```python
from build123d import *

# Parameters (mm, degrees)
SKIZZE1_W                       = 135
SKIZZE1_H                       = 135
SKIZZE1_W_2                     = 131
SKIZZE1_H_2                     = 131
AUFSATZ_LINEAR_AUSTRAGEN1_DEPTH = 18
SKIZZE2_W                       = 135
SKIZZE2_H                       = 135
AUFSATZ_LINEAR_AUSTRAGEN2_DEPTH = 5
SCHNITT_LINEAR_AUSTRAGEN1_DEPTH = 11
SKIZZE4_R                       = 1.75
SKIZZE4_R_2                     = 0.5
SCHNITT_LINEAR_AUSTRAGEN2_DEPTH = 10
FASE1_SIZE                      = 1


with BuildPart() as part:
    # Skizze1 → Aufsatz-Linear austragen1 (new body)
    with BuildSketch(Plane.XY):
        Rectangle(SKIZZE1_W, SKIZZE1_H)
        Rectangle(SKIZZE1_W_2, SKIZZE1_H_2, mode=Mode.SUBTRACT)
    extrude(amount=AUFSATZ_LINEAR_AUSTRAGEN1_DEPTH)

    # Skizze2 → Aufsatz-Linear austragen2 (add)
    with BuildSketch(Plane.XY.offset(18)):
        Rectangle(SKIZZE2_W, SKIZZE2_H)
    extrude(amount=AUFSATZ_LINEAR_AUSTRAGEN2_DEPTH)

    # Skizze3 → Schnitt-Linear austragen1 (cut)
    with BuildSketch(Plane.ZY.offset(67.5)):
        Polygon((5, -33.148996127), (3, -33.148996127), (3, -41.848996127), (5, -41.848996127), (7.4, -41.848996127), (7.4, -33.148996127), align=None)
    extrude(amount=-SCHNITT_LINEAR_AUSTRAGEN1_DEPTH, mode=Mode.SUBTRACT)

    # Skizze4 → Schnitt-Linear austragen2 (cut)
    with BuildSketch(Plane.XY.offset(23)):
        with BuildLine():
            Line((2.25, 56.5), (-2.25, 56.5))
            ThreePointArc((-2.25, 56.5), (-2.75, 56), (-2.25, 55.5))
            Line((-2.25, 55.5), (2.25, 55.5))
            ThreePointArc((2.25, 55.5), (2.75, 56), (2.25, 56.5))
        make_face()
        with BuildLine():
            Line((2.25, 58), (-2.25, 58))
            ThreePointArc((-2.25, 58), (-2.75, 57.5), (-2.25, 57))
            Line((-2.25, 57), (2.25, 57))
            ThreePointArc((2.25, 57), (2.75, 57.5), (2.25, 58))
        make_face()
        with BuildLine():
            Line((2.25, 59.5), (-2.25, 59.5))
            ThreePointArc((-2.25, 59.5), (-2.75, 59), (-2.25, 58.5))
            Line((-2.25, 58.5), (2.25, 58.5))
            ThreePointArc((2.25, 58.5), (2.75, 59), (2.25, 59.5))
        make_face()
        with Locations((0, 50)):
            Circle(SKIZZE4_R)
        with Locations((30, -50.5)):
            Circle(SKIZZE4_R)
        with Locations((10, -50.5)):
            Circle(SKIZZE4_R)
        with Locations((-10, -50.5)):
            Circle(SKIZZE4_R)
        with Locations((-30, -50.5)):
            Circle(SKIZZE4_R)
        with Locations((1, -56.5)):
            Circle(SKIZZE4_R_2)
        with Locations((1, -58.5)):
            Circle(SKIZZE4_R_2)
        with Locations((-1, -58.5)):
            Circle(SKIZZE4_R_2)
        with Locations((-1, -56.5)):
            Circle(SKIZZE4_R_2)
    extrude(amount=-SCHNITT_LINEAR_AUSTRAGEN2_DEPTH, mode=Mode.SUBTRACT)

    # Fase1
    fase1_edges = [part.edges().sort_by_distance(p)[0] for p in [
        (8.25, -50.5, 23),
        (-11.75, -50.5, 23),
        (-31.75, -50.5, 23),
        (28.25, -50.5, 23),
        (-1.75, 50, 23),
    ]]
    chamfer(fase1_edges, length=FASE1_SIZE)


solid = part.part
```
Can you work these out from the model? Positions are in its coordinate system, mm. A direction names the side the tool comes from. Coordinates: 2 decimals unless noted, no trailing zeros. Loops run counter-clockwise (first coordinate to the right, second up) from the corner with the lowest first, then second, coordinate; pieces in that order, holes last. Notation, with made-up numbers: (66.25, -15) - (77.25, -15) arc R23 cw to (77.25, 22) - close; hole circle Ø3 at (62.25, 82). An arc over 180 degrees is marked (long way). Use a Markdown table: item, result.
Item 1: We'd pull the mould along Y, two halves only. Please class faces 4 (the face through (-31.39, -51.56, 20.03)), 5 (the face through (0, 55.5, 21)), 6 (the face through (-1, -67.5, 11)), 7 (the face through (-1, 1, 23)): released by +Y, released by -Y, zero draft, split by the parting line, or undercut.
Numbers:
| item | result |
|---|---|
| face 4 | undercut |
| face 5 | undercut |
| face 6 | released by -Y |
| face 7 | zero draft |
Item 2: If I drill on probe 1 along X at (y, z) = (-58.5, 21.95); probe 2 along Y at (x, z) = (30, 19.8); probe 3 along X at (y, z) = (-28, 4.25), over which ranges is the centre line in solid material (lowest first)? Write a range as from..to.
Numbers:
| item | result |
|---|---|
| probe 1 | x = -67.5..-1.5, -0.5..0.5, 1.5..67.5 |
| probe 2 | y = -67.5..-52.25, -48.75..67.5 |
| probe 3 | x = -67.5..-65.5, 65.5..67.5 |
Item 3: I want a section at C-C on z = 11. Please give me the cut outline in (x, y), and give its area (3 significant figures).
Numbers:
| item | result |
|---|---|
| outline | (-67.5, -67.5) - (67.5, -67.5) - (67.5, 67.5) - (-67.5, 67.5) - close; hole (-65.5, -65.5) - (65.5, -65.5) - (65.5, 65.5) - (-65.5, 65.5) - close |
| area | 1,060 mm2 |
Item 4: For faces 1 (the face through (0, 59.5, 21)), 2 (the face through (-1, 67.5, 11)), 3 (the face through (-1, -65.5, 9)), which set-ups out of +Z, -Z, +X, -X, +Y, -Y let a thin tool reach every point of the face, with its end or its side?
Numbers:
| item | result |
|---|---|
| face 1 | +Z, -Z |
| face 2 | +Z, -Z, +X, -X, +Y |
| face 3 | -Z |
Item 5: Will these pins go through, and if not, where does the flat tip stop? pin 1 (12 mm diameter, centred on x = 52.5, y = -18.5, fed in from -Z); pin 2 (4 mm diameter, centred on x = 30, y = -50.5, fed in from +Z); pin 3 (3 mm diameter, centred on x = 10, y = -50.5, fed in from -Z).
Numbers:
| item | result |
|---|---|
| pin 1 | stops at z = 18 |
| pin 2 | stops at z = 22.25 |
| pin 3 | passes through |
Item 6: I want a section at D-D on x = 51. Please give me the cut outline in (y, z), and give its area (3 significant figures).
Numbers:
| item | result |
|---|---|
| outline | (-67.5, 0) - (-65.5, 0) - (-65.5, 18) - (65.5, 18) - (65.5, 0) - (67.5, 0) - (67.5, 23) - (-67.5, 23) - close |
| area | 747 mm2 |
Item 7: I want a section at A-A on y = 50. Please give me the cut outline in (x, z).
Numbers:
| item | result |
|---|---|
| outline | (-67.5, 0) - (-65.5, 0) - (-65.5, 18) - (-1.75, 18) - (-1.75, 22) - (-2.75, 23) - (-67.5, 23) - close; (1.75, 18) - (65.5, 18) - (65.5, 0) - (67.5, 0) - (67.5, 23) - (2.75, 23) - (1.75, 22) - close |
Item 8: I want a section at B-B on x = 30. Please give me the cut outline in (y, z), and give its area (4 significant figures).
Numbers:
| item | result |
|---|---|
| outline | (-67.5, 0) - (-65.5, 0) - (-65.5, 18) - (-52.25, 18) - (-52.25, 22) - (-53.25, 23) - (-67.5, 23) - close; (-48.75, 18) - (65.5, 18) - (65.5, 0) - (67.5, 0) - (67.5, 23) - (-47.75, 23) - (-48.75, 22) - close |
| area | 728.5 mm2 |
